```python
from build123d import *

# Parameters (mm, degrees)
CROQUIS3_R            = 5
CORTAR_EXTRUIR1_DEPTH = 51.41472999
MATRIZC1_COUNT        = 2
MATRIZC1_ANGLE        = 90


with BuildPart() as part:
    # Croquis1 → Revolución1 (revolve)
    with BuildSketch(Plane.XY, mode=Mode.PRIVATE) as revoluci_n1_sk:
        Polygon((-4, 0), (-4, 30), (-16.5, 30), (-16.5, 20), (-28.65, 20), (-28.65, 0), align=None)
    revolve(revoluci_n1_sk.sketch.rotate(Axis((0, 0, 0), (0, 1, 0)), 270), axis=Axis((0, 0, 0), (0, 1, 0)))

    # Croquis3 → Cortar-Extruir1 (cut, through all)
    with BuildSketch(Plane(origin=(0, 30, 0), x_dir=(1, 0, 0), z_dir=(0, 1, 0))):
        with Locations(Location((0, 0, 0), (0, 0, 270))):
            Circle(CROQUIS3_R)
    extrude(amount=-CORTAR_EXTRUIR1_DEPTH, mode=Mode.SUBTRACT)

    # Croquis6 → Taladro roscado M6x1.01 (revolve, cut)
    with BuildSketch(Plane(origin=(16.5, 25, 0), x_dir=(0, 0, -1), z_dir=(0, 1, 0))):
        Polygon((0, 0), (0, 18.502151548), (2.5, 17), (2.5, 0), align=None)
    taladro_roscado_m6x1_01 = revolve(axis=Axis((22.85, 25, 0), (-1, 0, 0)), mode=Mode.SUBTRACT)

    # MatrizC1: Taladro roscado M6x1.01 ×2 about axis
    matrizc1_axis = Axis((0, 30, 0), (0, -1, 0))
    for i in range(1, MATRIZC1_COUNT):
        add(taladro_roscado_m6x1_01.rotate(matrizc1_axis, i * MATRIZC1_ANGLE / (MATRIZC1_COUNT - 1)), mode=Mode.SUBTRACT)


solid = part.part
```
Here's how the part is built. I have some questions about the finished solid (model axes, mm). A direction names the side the tool comes from. Coordinates: 2 decimals unless noted, no trailing zeros. Loops run counter-clockwise (first coordinate to the right, second up) from the corner with the lowest first, then second, coordinate; pieces in that order, holes last. Notation, with made-up numbers: (13.25, 61) -> (55.25, 61) arc R11 ccw to (55.25, 74) -> close; hole circle Ø11 at (31, 5.5). An arc over 180 degrees is marked (long way). Return JSON: item names as keys, results as strings.
1) If we section it at B-B, the plane y = 23.5: Write out the boundary of the cut face in (x, z), then the cut area to 3 significant figures.
Results below:
{"outline": "(-2, 4.58) -> (-2, 16.38) arc R16.5 ccw (long way) to (16.38, -2) -> (4.58, -2) arc R5 cw (long way) to start; (2, 4.58) arc R5 cw to (4.58, 2) -> (16.38, 2) arc R16.5 ccw to (2, 16.38) -> close", "area": "684 mm²"}
2) Thinking about a two-plate mould opening in Y: for faces 4 (the face through (-0.33, 22.52, 10.5)), 5 (the face through (0, 0, -6)), 6 (the face through (3.4, 30, -3.9)), which applies, +Y half, -Y half, draft (parallel to the pull), parting line (faces both ways), or undercut?
Results below:
{"face 4": "undercut", "face 5": "-Y half", "face 6": "+Y half"}
3) For faces 1 (the face through (6.32, 24.93, -15.24)), 2 (the face through (-28.406, 9.86, 3.73)), 3 (the face through (10.5, 22.52, 0.33)), which set-ups out of +Z, -Z, +X, -X, +Y, -Y let a thin tool reach every point of the face, with its end or its side?
Results below:
{"face 1": "+Y", "face 2": "+Y, -Y", "face 3": "+X"}
4) Will these pins go through, and if not, where does the flat tip stop? pin 1 (2 mm diameter, centred on x = 17.5, y = 7.5, fed in from +Z); pin 2 (1 mm diameter, centred on y = 13, z = 7, fed in from +X); pin 3 (5 mm diameter, centred on x = 17.5, z = 19.5, fed in from +Y); pin 4 (9 mm diameter, centred on x = 0, z = 0, fed in from -Y).
Results below:
{"pin 1": "z = 23.42", "pin 2": "x = 27.9", "pin 3": "y = 20", "pin 4": "through"}
5) If we section it at D-D, the plane y = 16: Write out the boundary of the cut face in (x, z), then the cut area to 3 significant figures.
Results below:
{"outline": "circle Ø57.3 at (0, 0); hole circle Ø10 at (0, 0)", "area": "2,500 mm²"}
6) If we section it at A-A, the plane x = 0: Write out the boundary of the cut face in (y, z).
Results below:
{"outline": "(0, -28.65) -> (20, -28.65) -> (20, -16.5) -> (30, -16.5) -> (30, -5) -> (0, -5) -> close; (0, 5) -> (22.5, 5) -> (22.5, 16.5) -> (20, 16.5) -> (20, 28.65) -> (0, 28.65) -> close; (27.5, 5) -> (30, 5) -> (30, 16.5) -> (27.5, 16.5) -> close"}
7) I need wall thicknesses on line 1 (Y direction, x = 0, z = 8.25); line 2 (X direction, y = 18, z = 0); line 3 (X direction, y = 22, z = 0). Which ranges of each line are inside material? Lowest first, please. Write a range as from..to.
Results below:
{"line 1": "0..22.5, 27.5..30", "line 2": "-28.65..-5, 5..28.65", "line 3": "-16.5..-5, 5..16.5"}
8) If we section it at C-C, the plane z = 0: Write out the boundary of the cut face in (x, y).
Results below:
{"outline": "(-28.65, 0) -> (-5, 0) -> (-5, 30) -> (-16.5, 30) -> (-16.5, 20) -> (-28.65, 20) -> close; (5, 0) -> (28.65, 0) -> (28.65, 20) -> (16.5, 20) -> (16.5, 22.5) -> (5, 22.5) -> close; (5, 27.5) -> (16.5, 27.5) -> (16.5, 30) -> (5, 30) -> close"}
